from build123d import *

# Parameters (mm, degrees)
BOSS_EXTRUDE1_DEPTH = 101.6
SKETCH2_W           = 5.08
SKETCH2_H           = 6.35
BOSS_EXTRUDE2_DEPTH = 2.54
BOSS_EXTRUDE3_START = -101.6
SKETCH2_2_W         = 5.08
SKETCH2_2_H         = 6.35
BOSS_EXTRUDE3_DEPTH = 2.54
BOSS_EXTRUDE4_DEPTH = 1.524


with BuildPart() as part:
    # Sketch1 → Boss-Extrude1 (new body)
    with BuildSketch(Plane.XY):
        Polygon((0, 0), (38.1, 38.770841672), (38.1, 0), align=None)
    extrude(amount=BOSS_EXTRUDE1_DEPTH)

    # Sketch2 → Boss-Extrude2 (add)
    with BuildSketch(Plane.XY.offset(101.6)):
        with Locations((33.02, 26.035)):
            Rectangle(SKETCH2_W, SKETCH2_H)
    extrude(amount=BOSS_EXTRUDE2_DEPTH)

    # Sketch2<2> → Boss-Extrude3 (add)
    with BuildSketch(Plane.XY.offset(101.6).offset(BOSS_EXTRUDE3_START)):
        with Locations((33.02, 26.035)):
            Rectangle(SKETCH2_2_W, SKETCH2_2_H)
    extrude(amount=-BOSS_EXTRUDE3_DEPTH)

    # Sketch3 → Boss-Extrude4 (add)
    with BuildSketch(Plane(origin=(0, 0, 0), x_dir=(0, 0, 1), z_dir=(-0.7132504491541779, 0.7009092642998548, 0))):
        Polygon((12.7, 0), (12.7, 25.4), (38.1, 25.4), (38.1, 0), (40.64, 0), (40.64, 27.94), (10.16, 27.94), (10.16, 0), align=None)
        Polygon((88.9, 0), (88.9, 25.4), (63.5, 25.4), (63.5, 0), (60.96, 0), (60.96, 27.94), (91.44, 27.94), (91.44, 0), align=None)
    extrude(amount=BOSS_EXTRUDE4_DEPTH)


solid = part.part
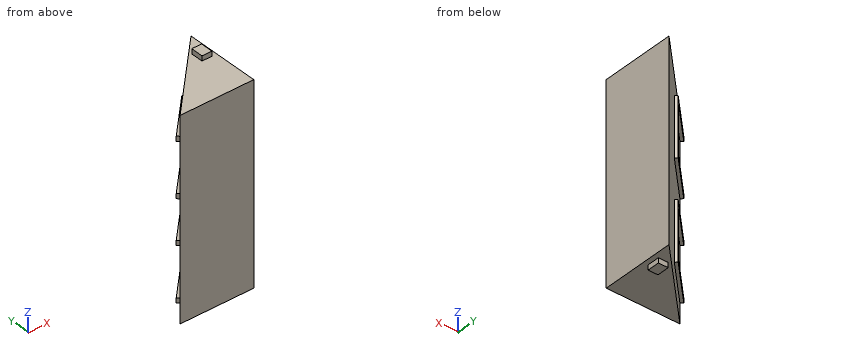
Verification items for the finished model (mm, model axes). Give positions to 0.01 mm unless a question says otherwise; leave off trailing zeros. Write each loop counter-clockwise with the first axis right and the second up, starting at its lowest first coordinate (ties: lowest second). Pieces come first, ordered by that corner, then holes. Notation, with made-up numbers: (77.25, -34.5) -> (81.25, -34.5) arc R24 ccw to (81.25, -18.5) -> close; hole circle Ø6 at (27, -39). An arc over 180 degrees is marked (long way). Use CSV: the item, a comma, the result in double quotes.
(1) Sectioned sample at A-A (z = 77). Record the cut outline in (x, y), plus the area to 3 significant figures.
Derived:
outline,"(0, 0) -> (38.1, 0) -> (38.1, 38.77) -> (19.58, 19.93) -> (18.5, 21) -> (16.72, 19.18) -> (17.8, 18.12) -> close"
area,"742 mm^2"
(2) Sectioned sample at D-D (x = 34). Record the cut outline in (y, z), plus the area to 3 significant figures.
Derived:
outline,"(0, 0) -> (22.86, 0) -> (22.86, -2.54) -> (29.21, -2.54) -> (29.21, 0) -> (34.6, 0) -> (34.6, 101.6) -> (29.21, 101.6) -> (29.21, 104.14) -> (22.86, 104.14) -> (22.86, 101.6) -> (0, 101.6) -> close"
area,"3,550 mm^2"
(3) Material ranges on L1, parallel to X at y = 31, z = 68; L2, parallel to Z at x = 5, y = 2; L3, parallel to Y at x = 17.5, z = 21, recorded low to high.
Derived:
L1,"x = 30.46 to 38.1"
L2,"z = 0 to 101.6"
L3,"y = 0 to 17.81, 18.41 to 19.98"
(4) Go/stop test with flat-tipped pins: pin 1 (12 mm diameter, centred on x = 11.5, y = 19.5, fed in from +Z); pin 2 (0.8 mm diameter, centred on x = 34, z = -0.5, fed in from -Y); pin 3 (5 mm diameter, centred on y = 16.5, z = 41, fed in from -X); pin 4 (12 mm diameter, centred on x = 23, z = 32, fed in from -Y). Record where each tip stops, or that it passes through.
Derived:
pin 1,"stops at z = 101.6"
pin 2,"stops at y = 22.86"
pin 3,"stops at x = 11.65"
pin 4,"stops at y = 0"
(5) Sectioned sample at B-B (y = 9). Record the cut outline in (x, z).
Derived:
outline,"(6.71, 10.16) -> (8.84, 10.16) -> (8.84, 0) -> (38.1, 0) -> (38.1, 101.6) -> (8.84, 101.6) -> (8.84, 91.44) -> (6.71, 91.44) -> (6.71, 88.9) -> (8.84, 88.9) -> (8.84, 63.5) -> (6.71, 63.5) -> (6.71, 60.96) -> (8.84, 60.96) -> (8.84, 40.64) -> (6.71, 40.64) -> (6.71, 38.1) -> (8.84, 38.1) -> (8.84, 12.7) -> (6.71, 12.7) -> close"
(6) Sectioned sample at C-C (x = 15). Record the cut outline in (y, z), plus the area to 3 significant figures.
Derived:
outline,"(0, 0) -> (15.26, 0) -> (15.26, 10.16) -> (17.44, 10.16) -> (17.44, 12.7) -> (15.26, 12.7) -> (15.26, 38.1) -> (17.44, 38.1) -> (17.44, 40.64) -> (15.26, 40.64) -> (15.26, 60.96) -> (17.44, 60.96) -> (17.44, 63.5) -> (15.26, 63.5) -> (15.26, 88.9) -> (17.44, 88.9) -> (17.44, 91.44) -> (15.26, 91.44) -> (15.26, 101.6) -> (0, 101.6) -> close"
area,"1,570 mm^2"
